Geometry check sheet. Reference: the model listing, model coordinates, mm. Face numbers are marked on the shaded views. A direction names the side the tool comes from. Coordinates: 2 decimals unless noted, no trailing zeros. Write each loop counter-clockwise with the first axis right and the second up, starting at its lowest first coordinate (ties: lowest second). Pieces come first, ordered by that corner, then holes. Notation, with made-up numbers: (22, 31.25) -> (54, 31.25) arc R20 ccw to (54, 53.25) -> close; hole circle Ø9 at (82.25, 62). An arc over 180 degrees is marked (long way). Answer in a Markdown table with one row per item. Add a question column.
Q1. Tool access check on the marked faces 1, 2 and 3. Record the directions out of +Z, -Z, +X, -X, +Y, -Y that give a thin tool (end or side, any length) a straight path to the whole face; none if there is none.
Q2. Section check D-D, the plane y = 0. Count the separate pieces of the cut face and the enclosed holes in it, and give its area (3 significant figures).
Q3. Thickness scan on line 1 (Y direction, x = 257.75, z = 0); line 2 (Y direction, x = 252.75, z = 56.5); line 3 (Y direction, x = 271, z = 0). Record the ranges inside material, lowest first.
Q4. Section check C-C, the plane x = 147. Record the boundary of the cut face in (y, z).
Q5. Release check for a two-part mould opening along Y. For the marked faces 4, 5 and 6 record: pulls with the +Y half, pulls with the -Y half, needs draft (parallel to the pull), parting line crosses it, or undercut.
Q6. Gauge pin test, flat ends, axial feed: P1, Ø1, axis at y = -48.5, z = -46.5, coming from the -X side; P2, Ø12, axis at x = 125.5, z = -28.5, coming from the +Y side; P3, Ø22, axis at y = -56.5, z = 97.86, coming from the +X side; P4, Ø12, axis at y = -96, z = -22, coming from the +X side. Record the tip position at first contact, or that the pin passes through.
Q7. Section check A-A, the plane z = -113. Record the boundary of the cut face in (x, y).
```python
from build123d import *

# Parameters (mm, degrees)
SKETCH_3_R           = 9.5
CUT_EXTRUDE_1_DEPTH  = 328.171973127
SKETCH_4_R           = 9.5
CUT_EXTRUDE_2_DEPTH  = 328.171973127
SKETCH_5_R           = 9.5
CUT_EXTRUDE_3_DEPTH  = 328.171973127
SKETCH_6_R           = 9.5
CUT_EXTRUDE_4_DEPTH  = 328.171973127
SKETCH_7_R           = 9.5
CUT_EXTRUDE_5_DEPTH  = 328.171973127
SKETCH_8_R           = 9.5
CUT_EXTRUDE_6_DEPTH  = 328.171973127
SKETCH_9_R           = 9.5
CUT_EXTRUDE_7_DEPTH  = 328.171973127
SKETCH_10_R          = 9.5
CUT_EXTRUDE_8_DEPTH  = 328.171973127
SKETCH_11_R          = 9.5
CUT_EXTRUDE_9_DEPTH  = 328.171973127
SKETCH_12_R          = 9.5
CUT_EXTRUDE_10_DEPTH = 328.171973127
SKETCH_13_R          = 9.5
CUT_EXTRUDE_11_DEPTH = 328.171973127
SKETCH_14_R          = 9.5
CUT_EXTRUDE_12_DEPTH = 328.171973127


with BuildPart() as part:
    # Эскиз1 → Повернуть1 (revolve)
    with BuildSketch(Plane.XY, mode=Mode.PRIVATE) as revolve_1_sk:
        Polygon((0, 0), (273, 0), (273, 98.4), (271.4, 100), (265, 100), (265, 127.5), (247, 127.5), (247, 100), (239, 100), (239, 62.5), (215, 62.5), (215, 55), (183, 55), (178.669872981, 52.5), (95, 52.5), (95, 50), (42, 50), (42, 45), (0, 45), align=None)
    revolve(revolve_1_sk.sketch.rotate(Axis((0, 0, 0), (1, 0, 0)), 90), axis=Axis((0, 0, 0), (1, 0, 0)))

    # Эскиз2 → Вырез-Повернуть1 (revolve, cut)
    with BuildSketch(Plane.XY, mode=Mode.PRIVATE) as cut_revolve_1_sk:
        Polygon((0, 0), (273, 0), (273, 95), (265, 95), (265, 45), (254, 45), (254, 39), (240, 39), (240, 34), (203.5, 34), (203.5, 31), (0, 31), align=None)
    revolve(cut_revolve_1_sk.sketch.rotate(Axis((0, 0, 0), (1, 0, 0)), 90), axis=Axis((0, 0, 0), (1, 0, 0)), mode=Mode.SUBTRACT)

    # Эскиз3 → Вырез-Вытянуть1 (cut, through all)
    with BuildSketch(Plane(origin=(0, 0, 0), x_dir=(0, 0, -1), z_dir=(1, 0, 0))):
        with Locations(Location((0, 113, 0), (0, 0, 180))):
            Circle(SKETCH_3_R)
    extrude(amount=CUT_EXTRUDE_1_DEPTH, mode=Mode.SUBTRACT)

    # Эскиз4 → Вырез-Вытянуть2 (cut, through all)
    with BuildSketch(Plane(origin=(0, 0, 0), x_dir=(0, 0, -1), z_dir=(1, 0, 0))):
        with Locations(Location((-56.5, 97.860870628, 0), (0, 0, 180))):
            Circle(SKETCH_4_R)
    extrude(amount=CUT_EXTRUDE_2_DEPTH, mode=Mode.SUBTRACT)

    # Эскиз5 → Вырез-Вытянуть3 (cut, through all)
    with BuildSketch(Plane(origin=(0, 0, 0), x_dir=(0, 0, -1), z_dir=(1, 0, 0))):
        with Locations(Location((-97.860870628, 56.5, 0), (0, 0, 180))):
            Circle(SKETCH_5_R)
    extrude(amount=CUT_EXTRUDE_3_DEPTH, mode=Mode.SUBTRACT)

    # Эскиз6 → Вырез-Вытянуть4 (cut, through all)
    with BuildSketch(Plane(origin=(0, 0, 0), x_dir=(0, 0, -1), z_dir=(1, 0, 0))):
        with Locations(Location((-113, 0, 0), (0, 0, 180))):
            Circle(SKETCH_6_R)
    extrude(amount=CUT_EXTRUDE_4_DEPTH, mode=Mode.SUBTRACT)

    # Эскиз7 → Вырез-Вытянуть5 (cut, through all)
    with BuildSketch(Plane(origin=(0, 0, 0), x_dir=(0, 0, -1), z_dir=(1, 0, 0))):
        with Locations(Location((-97.860870628, -56.5, 0), (0, 0, 180))):
            Circle(SKETCH_7_R)
    extrude(amount=CUT_EXTRUDE_5_DEPTH, mode=Mode.SUBTRACT)

    # Эскиз8 → Вырез-Вытянуть6 (cut, through all)
    with BuildSketch(Plane(origin=(0, 0, 0), x_dir=(0, 0, -1), z_dir=(1, 0, 0))):
        with Locations(Location((-56.5, -97.860870628, 0), (0, 0, 180))):
            Circle(SKETCH_8_R)
    extrude(amount=CUT_EXTRUDE_6_DEPTH, mode=Mode.SUBTRACT)

    # Эскиз9 → Вырез-Вытянуть7 (cut, through all)
    with BuildSketch(Plane(origin=(0, 0, 0), x_dir=(0, 0, -1), z_dir=(1, 0, 0))):
        with Locations(Location((0, -113, 0), (0, 0, 180))):
            Circle(SKETCH_9_R)
    extrude(amount=CUT_EXTRUDE_7_DEPTH, mode=Mode.SUBTRACT)

    # Эскиз10 → Вырез-Вытянуть8 (cut, through all)
    with BuildSketch(Plane(origin=(0, 0, 0), x_dir=(0, 0, -1), z_dir=(1, 0, 0))):
        with Locations(Location((56.5, -97.860870628, 0), (0, 0, 180))):
            Circle(SKETCH_10_R)
    extrude(amount=CUT_EXTRUDE_8_DEPTH, mode=Mode.SUBTRACT)

    # Эскиз11 → Вырез-Вытянуть9 (cut, through all)
    with BuildSketch(Plane(origin=(0, 0, 0), x_dir=(0, 0, -1), z_dir=(1, 0, 0))):
        with Locations(Location((97.860870628, -56.5, 0), (0, 0, 180))):
            Circle(SKETCH_11_R)
    extrude(amount=CUT_EXTRUDE_9_DEPTH, mode=Mode.SUBTRACT)

    # Эскиз12 → Вырез-Вытянуть10 (cut, through all)
    with BuildSketch(Plane(origin=(0, 0, 0), x_dir=(0, 0, -1), z_dir=(1, 0, 0))):
        with Locations(Location((113, 0, 0), (0, 0, 180))):
            Circle(SKETCH_12_R)
    extrude(amount=CUT_EXTRUDE_10_DEPTH, mode=Mode.SUBTRACT)

    # Эскиз13 → Вырез-Вытянуть11 (cut, through all)
    with BuildSketch(Plane(origin=(0, 0, 0), x_dir=(0, 0, -1), z_dir=(1, 0, 0))):
        with Locations(Location((97.860870628, 56.5, 0), (0, 0, 180))):
            Circle(SKETCH_13_R)
    extrude(amount=CUT_EXTRUDE_11_DEPTH, mode=Mode.SUBTRACT)

    # Эскиз14 → Вырез-Вытянуть12 (cut, through all)
    with BuildSketch(Plane(origin=(0, 0, 0), x_dir=(0, 0, -1), z_dir=(1, 0, 0))):
        with Locations(Location((56.5, 97.860870628, 0), (0, 0, 180))):
            Circle(SKETCH_14_R)
    extrude(amount=CUT_EXTRUDE_12_DEPTH, mode=Mode.SUBTRACT)


solid = part.part
```
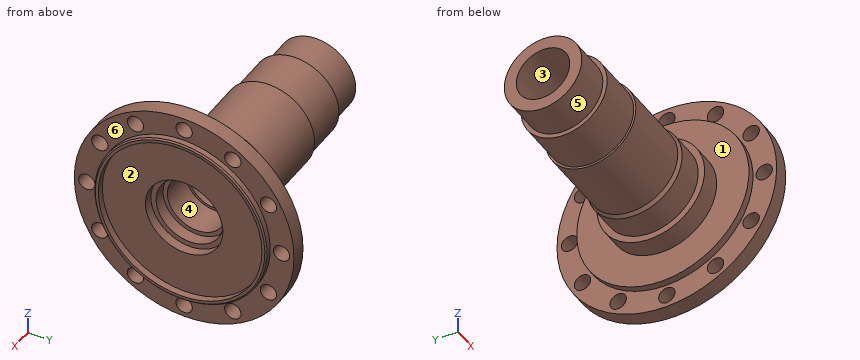
Calculated:
| question | item | result |
|---|---|---|
| 1 | face 1 | -X |
| 1 | face 2 | +X |
| 1 | face 3 | +X, -X |
| 2 | separate pieces | 4 |
| 2 | enclosed holes | 0 |
| 2 | area | 13,300 mm² |
| 3 | line 1 | y = -127.5 to -122.5, -103.5 to -45, 45 to 103.5, 122.5 to 127.5 |
| 3 | line 2 | y = -114.3 to -107.36, -88.36 to 88.36, 107.36 to 114.3 |
| 3 | line 3 | y = -100 to -95, 95 to 100 |
| 4 | outline | circle Ø105 at (0, 0); hole circle Ø62 at (0, 0) |
| 5 | face 4 | undercut |
| 5 | face 5 | parting line crosses it |
| 5 | face 6 | needs draft |
| 6 | P1 | stops at x = 239 |
| 6 | P2 | stops at y = 47.43 |
| 6 | P3 | stops at x = 265 |
| 6 | P4 | stops at x = 273 |
| 7 | outline | (247, -59.05) -> (265, -59.05) -> (265, -9.5) -> (247, -9.5) -> close; (247, 9.5) -> (265, 9.5) -> (265, 59.05) -> (247, 59.05) -> close |
